Could you check a few things on this model? Use its own coordinates, in mm. Face numbers are marked on the shaded views. A direction names the side the tool comes from. Round coordinates to 2 decimals unless told otherwise and drop trailing zeros. Loops run counter-clockwise (first coordinate to the right, second up) from the corner with the lowest first, then second, coordinate; pieces in that order, holes last.
from build123d import *

# Parameters (mm, degrees)
BOSS_EXTRUDE1_DEPTH      = 1.5875
BOSS_EXTRUDE3_DEPTH      = 120
BOSS_EXTRUDE3_DEPTH_BACK = 120
CUT_EXTRUDE1_DEPTH       = 182.234838864


with BuildPart() as part:
    # Sketch1 → Boss-Extrude1 (new body)
    with BuildSketch(Plane.XY):
        Polygon((-55.589527783, -99.278633486), (-123.629375351, -95.224778061), (-9.287976323, 89.663408039), (24.731947461, 30.599888109), (-15.428790161, -34.339372689), align=None)
    extrude(amount=BOSS_EXTRUDE1_DEPTH)

    # Sketch4 → Boss-Extrude3 (add, two sides: drawn at the far end of the back side and taken through both)
    with BuildSketch(Plane(origin=(-19.629912529, -31.741249903, 0), x_dir=(0.8504980945941722, -0.5259781279594072, 0), z_dir=(0.5259781279594072, 0.8504980945941724, 0)).offset(-BOSS_EXTRUDE3_DEPTH_BACK)):
        with BuildLine():
            Line((-55.060397672, -1.5875), (-55.060397672, 0))
            add(Edge.make_bspline(
                [(-55.060397672, 0), (-65.213115138, 0), (-72.548531989, -8.632316441)],
                knots=[0.320978727, 0.320978727, 0.320978727, 1.185471829, 1.185471829, 1.185471829], degree=2, weights=[1, 0.908026935, 1]))
            ThreePointArc((-72.548531989, -8.632316441), (-72.721094469, -8.860608628), (-72.890676993, -9.091123051))
            Line((-72.890676993, -9.091123051), (-72.745996539, -9.14666735))
            Line((-72.745996539, -9.14666735), (-71.891585739, -9.474684354))
            add(Edge.make_bspline(
                [(-55.060397672, -1.5875), (-64.677105487, -1.5875), (-71.891585739, -9.474684354)],
                knots=[3.462571381, 3.462571381, 3.462571381, 4.286530008, 4.286530008, 4.286530008], degree=2, weights=[1, 0.916330054, 1]))
        make_face()
    extrude(amount=BOSS_EXTRUDE3_DEPTH + BOSS_EXTRUDE3_DEPTH_BACK)

    # Sketch5 → Cut-Extrude1 (cut, through all)
    with BuildSketch(Plane(origin=(0, 0, 0), x_dir=(-1, 0, 0), z_dir=(0, 0, -1))):
        Polygon((9.287976323, 89.663408039), (21.860519309, 111.491165443), (10.387842561, 118.099298331), (-2.424711001, 95.854847771), align=None)
        Polygon((123.629375351, -95.224778061), (148.774461323, -93.726618573), (149.561894462, -106.94288435), (123.936787337, -108.46964379), align=None)
    extrude(amount=-CUT_EXTRUDE1_DEPTH, mode=Mode.SUBTRACT)


solid = part.part
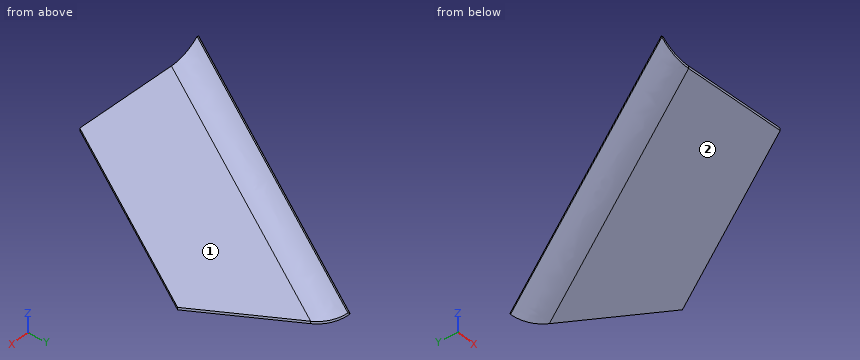
Item 1: If I drill on line 1 along Z through (x, y) = (-53.5, -37); line 2 along Y through (x, z) = (-38, 6.75); line 3 along X through (y, z) = (50.5, 5.75), over which ranges is the centre line in solid material (lowest first)?
Results list:
line 1: z = 0 to 1.59
line 2: y = 69.73 to 73.14
line 3: x = -50.72 to -48.33
Item 2: For the marked faces 1 and 2, which set-ups out of +Z, -Z, +X, -X, +Y, -Y let a thin tool reach every point of the face, with its end or its side?
Results list:
face 1: +Z, +X, -Y
face 2: -Z, +X, -X, +Y, -Y
Item 3: If we section it at B-B, the plane x = -5.5: Please give me the cut outline in (y, z), then the cut area to 3 significant figures.
Results list:
outline: (-18.28, 0) - (83.09, 0) - (83.09, 1.59) - (-18.28, 1.59) - close
area: 161 mm2
Item 4: If we section it at A-A, the plane x = 12: Please give me the cut outline in (y, z), then the cut area to 3 significant figures.
Results list:
outline: (10.01, 0) - (52.7, 0) - (52.7, 1.59) - (10.01, 1.59) - close
area: 67.8 mm2
Item 5: Will these pins go through, and if not, where does the flat tip stop? pin 1 (3 mm diameter, centred on y = 62.5, z = 8.5, fed in from +X); pin 2 (4 mm diameter, centred on x = -19, y = 81, fed in from +Z); pin 3 (1 mm diameter, centred on x = -59, y = 11, fed in from +Z).
Results list:
pin 1: stops at x = -42.64
pin 2: stops at z = 2.41
pin 3: stops at z = 1.64
